from build123d import *

# Parameters (mm, degrees)
SALIENTE_EXTRUIR1_DEPTH = 45
VACIADO1_T              = -3


with BuildPart() as part:
    # Croquis1 → Saliente-Extruir1 (new body)
    with BuildSketch(Plane(origin=(0, 0, 0), x_dir=(0, 0, -1), z_dir=(1, 0, 0))):
        Polygon((0, 0), (27, 10), (27, 0), align=None)
    extrude(amount=SALIENTE_EXTRUIR1_DEPTH)

    # Vaciado1
    vaciado1_openings = [part.faces().sort_by_distance(p)[0] for p in [
        (22.5, 5, -13.5),
    ]]
    offset(amount=VACIADO1_T, openings=vaciado1_openings, kind=Kind.INTERSECTION)


solid = part.part
The model under review builds one solid part; all positions refer to its coordinate system, in mm. A direction names the side the tool comes from. Round coordinates to 2 decimals unless told otherwise and drop trailing zeros. Write each loop counter-clockwise with the first axis right and the second up, starting at its lowest first coordinate (ties: lowest second). Pieces come first, ordered by that corner, then holes. Notation, with made-up numbers: M 63,21 L 81,21 A28 ccw 81,53 Z; hole C -23.5,-32 d9. An arc over 180 degrees is marked long. Answer as CSV lines item,"result". Start each with the question number.
Q1. Consider section B-B, the plane x = 7. Give the boundary of the cut face in (y, z), then the cut area to 3 significant figures.
Q2. Consider section C-C, the plane z = -16.75. Give the boundary of the cut face in (x, y).
Q3. The part is to be moulded in two halves that separate along X. For faces 1 (the face through (45, 3, -20)), 2 (the face through (22, 0, -14)), 3 (the face through (22, 3, -16)), say which applies: +X half, -X half, draft (parallel to the pull), parting line (faces both ways), or undercut.
Q4. Wall thickness on line 1 along Y through (x, z) = (31, -17); line 2 along X through (y, z) = (4.25, -16.5); line 3 along Z through (x, y) = (5, 8.5): over which ranges is each line inside the solid? List them lowest first.
Q5. Consider section A-A, the plane y = 4.5. Give the boundary of the cut face in (x, z), then the cut area to 3 significant figures.
Q6. Tool access review of faces 4 (the face through (3, 5, -20)), 5 (the face through (22, 5, -27)): name each direction out of +Z, -Z, +X, -X, +Y, -Y from which nothing blocks a thin tool from reaching the whole face with its end or side.
Q7. Consider section D-D, the plane y = 2. Give the boundary of the cut face in (x, z).
Q8. Clearance check with flat-ended pins moving along their axes: P1, Ø4.5, axis at x = 14, y = 5.5, coming from the +Z side; P2, Ø8, axis at x = 23, z = -15, coming from the +Y side; P3, Ø8, axis at x = 5, z = -6, coming from the -Y side. State where each tip first meets the part, or that it passes through.
Result set:
1,outline,"M 0,-27 L 10,-27 L 8.89,-24 L 3,-24 L 3,-8.1 L 0,0 Z"
1,area,"88.2 mm²"
2,outline,"M 0,0 L 45,0 L 45,6.2 L 42,6.2 L 42,3 L 3,3 L 3,6.2 L 0,6.2 Z"
3,face 1,"+X half"
3,face 2,"draft"
3,face 3,"undercut"
4,line 1,"y = 0 to 3"
4,line 2,"x = 0 to 3, 42 to 45"
4,line 3,"z = -27 to -24"
5,outline,"M 0,-27 L 45,-27 L 45,-12.15 L 42,-12.15 L 42,-24 L 3,-24 L 3,-12.15 L 0,-12.15 Z"
5,area,"206 mm²"
6,face 4,"+Z, +Y"
6,face 5,"-Z, +X, -X, +Y, -Y"
7,outline,"M 0,-27 L 45,-27 L 45,-5.4 L 0,-5.4 Z"
8,P1,"stops at z = -24"
8,P2,"stops at y = 3"
8,P3,"stops at y = 0"
